CAD build for the part. Positions are in the model's coordinates, mm. A direction names the side the tool comes from. Round coordinates to 2 decimals unless told otherwise and drop trailing zeros. Order: outer loops, then holes, each group sorted by start corner. A loop starts at its lowest first (then second) coordinate and runs counter-clockwise, first axis right, second up. Notation, with made-up numbers: (17, 58.5) - (68, 58.5) arc R9 ccw to (68, 65.5) - close; hole circle Ø8 at (53.5, 3). An arc over 180 degrees is marked (long way). Use one line per item in the form item = value. Start each with the question number.
from build123d import *

# Parameters (mm, degrees)
SKETCH1_W           = 126
SKETCH1_H           = 136
BOSS_EXTRUDE1_DEPTH = 3
SKETCH2_W           = 126
SKETCH2_H           = 136
SKETCH2_W_2         = 120
SKETCH2_H_2         = 130
BOSS_EXTRUDE2_DEPTH = 45
FILLET1_R           = 5
SKETCH4_W           = 82
SKETCH4_H           = 23
SKETCH4_W_2         = 50
SKETCH4_H_2         = 10
CUT_EXTRUDE1_DEPTH  = 10


with BuildPart() as part:
    # Sketch1 → Boss-Extrude1 (new body)
    with BuildSketch(Plane(origin=(0, 0, 0), x_dir=(1, 0, 0), z_dir=(0, 1, 0))):
        Rectangle(SKETCH1_W, SKETCH1_H)
    extrude(amount=BOSS_EXTRUDE1_DEPTH)

    # Sketch2 → Boss-Extrude2 (add)
    with BuildSketch(Plane(origin=(0, 3, 0), x_dir=(1, 0, 0), z_dir=(0, 1, 0))):
        Rectangle(SKETCH2_W, SKETCH2_H)
        Rectangle(SKETCH2_W_2, SKETCH2_H_2, mode=Mode.SUBTRACT)
    extrude(amount=BOSS_EXTRUDE2_DEPTH)

    # Fillet1
    fillet1_edges = [part.edges().sort_by_distance(p)[0] for p in [
        (63, 24, 68),
        (-63, 24, 68),
        (-63, 24, -68),
        (63, 24, -68),
    ]]
    fillet(fillet1_edges, radius=FILLET1_R)

    # Sketch4 → Cut-Extrude1 (cut)
    with BuildSketch(Plane(origin=(0, 3, 0), x_dir=(1, 0, 0), z_dir=(0, 1, 0))):
        with Locations((0, -20.828487482)):
            Rectangle(SKETCH4_W, SKETCH4_H)
        with Locations((0, 20.671512518)):
            Rectangle(SKETCH4_W_2, SKETCH4_H_2)
    extrude(amount=-CUT_EXTRUDE1_DEPTH, mode=Mode.SUBTRACT)


solid = part.part
(1) Slice it at A-A (x = 11). Give the cut face in (y, z), and give its area (3 significant figures).
(2) Slice it at B-B (x = 34). Give the cut face in (y, z), and give its area (3 significant figures).
(3) Wall check: line 1 (X direction, y = 11, z = -38); line 2 (Z direction, x = -38.5, y = 22.5); line 3 (Y direction, x = -39, z = 43). Give the ranges that are in metal, low to high. Write a range as [from, to].
(4) Slice it at D-D (z = -8.5). Give the cut face in (x, y).
(5) Which spindle directions (+Z, -Z, +X, -X, +Y, -Y) get a long thin tool onto all of the face, cutting with end or side? Do faces 4 (the flat face through (-60, 25, 1)), 5 (the cylindrical face through (-62, 24, -66)), 6 (the flat face through (0, 2, -25.672)). Say none if no direction does.
(6) Slice it at C-C (y = 9). Give the cut face in (x, z), and give its area (3 significant figures).
(7) Mould opens along Z. For faces 1 (the cylindrical face through (62, 24, -66)), 2 (the flat face through (-1, 3, -1)), 3 (the flat face through (-1, 24, 68)) say: pulls with the +Z half, pulls with the -Z half, needs draft (parallel to the pull), parting line crosses it, or undercut.
(8) Flat gauge pins, fed straight in: P1, Ø10, axis at x = -16.5, z = 44.5, coming from the +Y side; P2, Ø5, axis at x = 37, z = 0.5, coming from the -Y side. Where does each tip first touch, or does it go through?
Results list:
q1.outline = (0, -68) - (48, -68) - (48, -65) - (3, -65) - (3, -25.67) - (0, -25.67) - close; (0, -15.67) - (3, -15.67) - (3, 9.33) - (0, 9.33) - close; (0, 32.33) - (3, 32.33) - (3, 65) - (48, 65) - (48, 68) - (0, 68) - close
q1.area = 579 mm²
q2.outline = (0, -68) - (48, -68) - (48, -65) - (3, -65) - (3, 9.33) - (0, 9.33) - close; (0, 32.33) - (3, 32.33) - (3, 65) - (48, 65) - (48, 68) - (0, 68) - close
q2.area = 609 mm²
q3.line_1 = [-63, -60], [60, 63]
q3.line_2 = [-68, -65], [65, 68]
q3.line_3 = [0, 3]
q4.outline = (-63, 0) - (63, 0) - (63, 48) - (60, 48) - (60, 3) - (-60, 3) - (-60, 48) - (-63, 48) - close
q5.face_4 = +Y
q5.face_5 = -Z, -X, +Y, -Y
q5.face_6 = +Y, -Y
q6.outline = (-63, -63) arc R5 ccw to (-58, -68) - (58, -68) arc R5 ccw to (63, -63) - (63, 63) arc R5 ccw to (58, 68) - (-58, 68) arc R5 ccw to (-63, 63) - close; hole (-60, -65) - (60, -65) - (60, 65) - (-60, 65) - close
q6.area = 1,510 mm²
q7.face_1 = pulls with the -Z half
q7.face_2 = undercut
q7.face_3 = pulls with the +Z half
q8.P1 = 3
q8.P2 = 0
